```python
from build123d import *

# Parameters (mm, degrees)
F0_W     = 76.2
F0_H     = 76.2
F1_DEPTH = 38.1
F2_W     = 19.05
F2_H     = 44.45
F3_DEPTH = 69.85
F5_DEPTH = 19.05


with BuildPart() as f1:
    # F0 (on Front) → F1 (new body)
    with BuildSketch(Plane.XZ):
        with Locations((-26.431875, 3.83165)):
            Rectangle(F0_W, F0_H)
    extrude(amount=F1_DEPTH)

    # F2 (on face) → F3 (join)
    with BuildSketch(Plane.YZ.offset(11.668125)):
        with Locations((-9.525, 3.83165)):
            Rectangle(F2_W, F2_H)
    extrude(amount=F3_DEPTH)

    # F4 (on face) → F5 (join)
    with BuildSketch(Plane.XZ.offset(19.05)):
        Polygon((81.518125, 41.93165), (11.668125, 26.05665), (81.518125, 26.05665), align=None)
        Polygon((81.518125, -18.39335), (11.668125, -18.39335), (81.518125, -34.26835), align=None)
    extrude(amount=-F5_DEPTH)


solid = f1.part
```
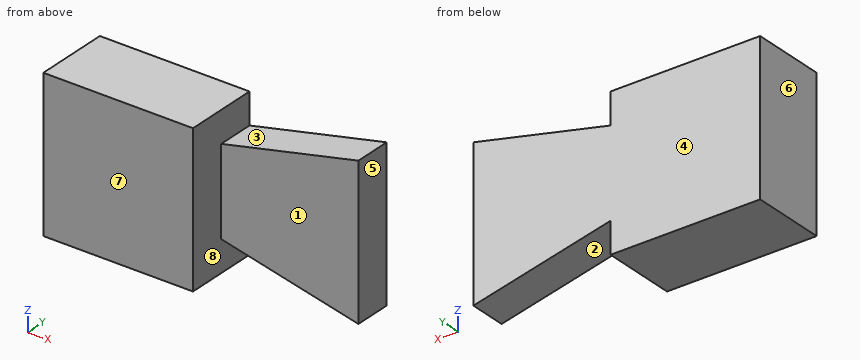
The listing builds one solid part. Answer for the finished solid, in the listing's coordinates (mm). Face numbers are marked on the shaded views. A direction names the side the tool comes from. Coordinates: 2 decimals unless noted, no trailing zeros. Write each loop counter-clockwise with the first axis right and the second up, starting at its lowest first coordinate (ties: lowest second). Pieces come first, ordered by that corner, then holes.
Q1. The mould has two halves that part along X. Classify the marked faces 6, 7 and 8: released by +X, released by -X, zero draft, split by the parting line, or undercut.
Returned:
face 6: released by -X
face 7: zero draft
face 8: undercut
Q2. Given P1, Ø2, axis at y = -29.5, z = 6.5, coming from the +X side, flat-ended and moving along its own axis, determine where the tip first touches the part or whether it passes through.
Returned:
P1: stops at x = 11.67
Q3. Which of the six approach directions +Z, -Z, +X, -X, +Y, -Y give full straight-line access (tool end or side, diameter ignored) to the marked faces 1, 2, 3, 4 and 5?
Returned:
face 1: +Z, -Z, +X, -Y
face 2: -Z, +Y, -Y
face 3: +Z, +Y, -Y
face 4: +Z, -Z, +X, -X, +Y
face 5: +Z, -Z, +X, +Y, -Y
Q4. Section B-B, the plane z = -28 is taken. Write down the section's boundary in (x, y).
Returned:
outline: (-64.53, -38.1) - (11.67, -38.1) - (11.67, 0) - (-64.53, 0) - close; (53.94, -19.05) - (81.52, -19.05) - (81.52, 0) - (53.94, 0) - close
Q5. Section C-C, the plane z = 18 is taken. Write down the section's boundary in (x, y).
Returned:
outline: (-64.53, -38.1) - (11.67, -38.1) - (11.67, -19.05) - (81.52, -19.05) - (81.52, 0) - (-64.53, 0) - close
Q6. Section A-A, the plane y = -2.5 is taken. Write down the section's boundary in (x, z).
Returned:
outline: (-64.53, -34.27) - (11.67, -34.27) - (11.67, -18.39) - (81.52, -34.27) - (81.52, 41.93) - (11.67, 26.06) - (11.67, 41.93) - (-64.53, 41.93) - close
Q7. Find the intervals of material crossed by line 1 along X through (y, z) = (-25, -21.5); line 2 along Y through (x, z) = (20, -13); line 3 along Z through (x, y) = (42, -11), in increasing order.
Returned:
line 1: x = -64.53 to 11.67
line 2: y = -19.05 to 0
line 3: z = -25.29 to 32.95
Q8. Section D-D, the plane x = 27 is taken. Write down the section's boundary in (y, z), then the cut area to 3 significant figures.
Returned:
outline: (-19.05, -21.88) - (0, -21.88) - (0, 29.54) - (-19.05, 29.54) - close
area: 980 mm2
